Autodesk Inventor part; units mm, degrees
ref_plane "YZ Plane" through (0, 0, 0) normal (1, 0, 0) x (0, 1, 0)
ref_plane "XZ Plane" through (0, 0, 0) normal (0, 1, 0) x (-1, 0, 0)
ref_plane "XY Plane" through (0, 0, 0) normal (0, 0, 1) x (1, 0, 0)
sketch "Sketch1" plane through (0, 0, 0) normal (0, 1, 0) x (-1, 0, 0)
  line L0 (0, 0) -> (381, 0)
  line L1 (381, 0) -> (381, -25.4)
  line L2 (381, -25.4) -> (0, -25.4)
  line L3 (0, -25.4) -> (0, 0)
  dimension "d0" = 381
  dimension "d1" = 25.4
extrude "Extrusion1" add sketch "Sketch1" along normal blind 3.429
sketch "Sketch2" plane through (0, 3.429, 0) normal (0, 1, 0) x (1, 0, 0)
  line L0 (0, 25.4) -> (-381, 25.4)
  line L1 (-50.8, 25.4) -> (-89.0524, 25.4)
  line L2 (-89.0524, 25.4) -> (-89.0524, 21.7932)
  line L3 (-89.0524, 21.7932) -> (-50.8, 21.7932)
  line L4 (-50.8, 21.7932) -> (-50.8, 25.4)
  line L5 (0, 0) -> (0, 25.4)
  line L6 (-127.1524, 25.4) -> (-257.6322, 25.4)
  line L7 (-257.6322, 25.4) -> (-257.6322, 21.7932)
  line L8 (-257.6322, 21.7932) -> (-127.1524, 21.7932)
  line L9 (-127.1524, 21.7932) -> (-127.1524, 25.4)
  point P0 (-89.0524, 23.5966)
  dimension "d4" = 38.2524
  dimension "d5" = 3.6068
  dimension "d6" = 50.8
  dimension "d7" = 38.1
  dimension "d8" = 3.6068
  dimension "d9" = 130.4798
extrude "Extrusion2" add sketch "Sketch2" along normal blind 12.5984
sketch "Sketch3" plane through (0, 16.0274, 0) normal (0, 1, 0) x (1, 0, 0)
  line L0 (-381, 25.4) -> (-381, 0)
  line L1 (-257.6322, 25.4) -> (-381, 25.4)
  line L2 (-381, 0) -> (0, 0)
  line L3 (0, 0) -> (0, 25.4)
  line L4 (0, 25.4) -> (-381, 25.4)
  line L5 (-381, 25.4) -> (-381, 0)
  line L6 (-381, 0) -> (0, 0)
  line L7 (0, 0) -> (0, 25.4)
extrude "Extrusion3" add sketch "Sketch3" along normal blind 3.429
sketch "Sketch5" plane through (0, 19.4564, 0) normal (0, 1, 0) x (1, 0, 0)
  line L0 (0, 0) -> (0, 25.4)
  line L1 (0, 25.4) -> (-381, 25.4)
  point P0 (-12.7, 12.7)
  point P1 (-245.745, 25.4)
  dimension "d18" = 12.7
  dimension "d19" = 12.7
hole "Hole1" at (-12.7, 19.4564, -12.7) direction (0, -1, 0) diameter 6.5024 end through all
sketch "Sketch6" plane through (0, 19.4564, 0) normal (0, 1, 0) x (1, 0, 0)
  line L0 (0, 25.4) -> (-381, 25.4)
  line L1 (-381, 25.4) -> (-381, 0)
  point P0 (-177.8, 12.7)
  point P1 (-245.745, 25.4)
  dimension "d36" = 12.7
  dimension "d37" = 203.2
hole "Hole2" at (-177.8, 19.4564, -12.7) direction (0, -1, 0) diameter 6.5024 end through all
sketch "Sketch7" plane through (0, 19.4564, 0) normal (0, 1, 0) x (1, 0, 0)
  line L0 (0, 25.4) -> (-381, 25.4)
  line L1 (-381, 25.4) -> (-381, 0)
  point P0 (0, 0)
  point P1 (-368.3, 12.7)
  point P2 (-279.654, 25.4)
  dimension "d38" = 12.7
  dimension "d39" = 12.7
hole "Hole3" at (-368.3, 19.4564, -12.7) direction (0, -1, 0) diameter 6.5024 end through all
sketch "Sketch10" plane through (0, 19.4564, 0) normal (0, 1, 0) x (1, 0, 0)
  line L0 (0, 25.4) -> (-381, 25.4)
  line L1 (0, 0) -> (0, 25.4)
  point P0 (-88.9, 12.7)
  point P1 (-245.745, 25.4)
  point P2 (0, 12.7)
  dimension "d64" = 12.7
  dimension "d74" = 88.9
hole "Hole6" at (-88.9, 19.4564, -12.7) direction (0, -1, 0) diameter 6.5024 end through all
ref_plane "Work Plane2" through (0, 9.7282, 0) normal (0, 1, 0) x (1, 0, 0)
sketch "Sketch11" plane through (0, 0, 0) normal (0, -1, 0) x (1, 0, 0)
  line L0 (-279.654, -25.4) -> (-279.654, -13.3858)
  line L1 (-279.654, -13.3858) -> (-245.745, -13.3858)
  line L2 (-245.745, -25.4) -> (-245.745, -13.3858)
  line L3 (-245.745, -13.3858) -> (-279.654, -13.3858)
  line L4 (-279.654, -13.3858) -> (-279.654, -25.4)
  line L5 (-279.654, -25.4) -> (-245.745, -25.4)
  line L6 (-245.745, -25.4) -> (-245.745, -13.3858)
  point P0 (0, 0)
extrude "Extrusion5" cut sketch "Sketch11" against normal blind 7.9375
properties part number "ArmPart1"
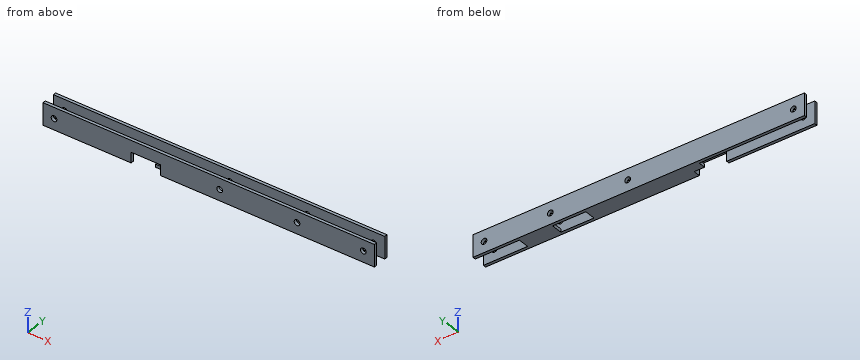
Input: part model. Units: mm. Frame: model coordinates. Give positions to 0.01 mm unless a question says otherwise; leave off trailing zeros. Write each loop counter-clockwise with the first axis right and the second up, starting at its lowest first coordinate (ties: lowest second). Pieces come first, ordered by that corner, then holes. Notation, with made-up numbers: (39.25, -1.75) - (43.25, -1.75) arc R20 ccw to (43.25, 2.25) - close; hole circle Ø9 at (-6, -15.5). An arc over 180 degrees is marked (long way). Write item = value, one per line. Start each with the question number.
1) Cut plane A-A (x = -263). Return loops of the section in (y, z), and give its area (3 significant figures).
2) Cut plane B-B (z = -3.5). Return loops of the section in (x, y).
3) Material intervals for L1, parallel to X at y = 17.8, z = -12.7; L2, parallel to Y at x = -16.5, z = -6.75; L3, parallel to Z at x = -177.8, y = 2.4, sorted ascending. Write a range as [from, to].
4) Pin query (flat end, axial travel): pin 1 (8.5 mm diameter, centred on x = -177.8, z = -12.7, fed in from +Y); pin 2 (4 mm diameter, centred on x = -175, y = 9, fed in from +Z); pin 3 (6 mm diameter, centred on y = 7.5, z = -19, fed in from +X); pin 4 (1.1 mm diameter, centred on y = 11, z = -23, fed in from -X). Return the tip coordinate at first contact, or that it passes through.
5) Cut plane C-C (x = -177.8). Return loops of the section in (y, z).
6) Cut plane D-D (x = -12.7). Return loops of the section in (y, z), and give its area (3 significant figures).
Answers follow:
q1.outline = (0, -13.39) - (3.43, -13.39) - (3.43, 0) - (0, 0) - close; (16.03, -25.4) - (19.46, -25.4) - (19.46, 0) - (16.03, 0) - close
q1.area = 133 mm^2
q2.outline = (-381, 0) - (0, 0) - (0, 3.43) - (-381, 3.43) - close; (-381, 16.03) - (0, 16.03) - (0, 19.46) - (-381, 19.46) - close
q3.L1 = [-381, -371.55], [-365.05, -181.05], [-174.55, -92.15], [-85.65, -15.95], [-9.45, 0]
q3.L2 = [0, 3.43], [16.03, 19.46]
q3.L3 = [-25.4, -15.95], [-9.45, 0]
q4.pin_1 = 19.46
q4.pin_2 = -21.79
q4.pin_3 = -50.8
q4.pin_4 = -257.63
q5.outline = (0, -25.4) - (19.46, -25.4) - (19.46, -15.95) - (16.03, -15.95) - (16.03, -21.79) - (3.43, -21.79) - (3.43, -15.95) - (0, -15.95) - close; (0, -9.45) - (3.43, -9.45) - (3.43, 0) - (0, 0) - close; (16.03, -9.45) - (19.46, -9.45) - (19.46, 0) - (16.03, 0) - close
q6.outline = (0, -25.4) - (3.43, -25.4) - (3.43, -15.95) - (0, -15.95) - close; (0, -9.45) - (3.43, -9.45) - (3.43, 0) - (0, 0) - close; (16.03, -25.4) - (19.46, -25.4) - (19.46, -15.95) - (16.03, -15.95) - close; (16.03, -9.45) - (19.46, -9.45) - (19.46, 0) - (16.03, 0) - close
q6.area = 130 mm^2
